The drawing under review shows one solid part. Ordinate dimensions are in mm from its lowest x, y, z. A direction names the side the tool comes from. Coordinates: 2 decimals unless noted, no trailing zeros. Order: outer loops, then holes, each group sorted by start corner. A loop starts at its lowest first (then second) coordinate and runs counter-clockwise, first axis right, second up. Notation, with made-up numbers: (65.5, 40.25) -> (84.5, 40.25) arc R24 ccw to (84.5, 55.25) -> close; hole circle Ø2 at (29.5, 48.5). An arc over 180 degrees is marked (long way). Write item = value, one per line.
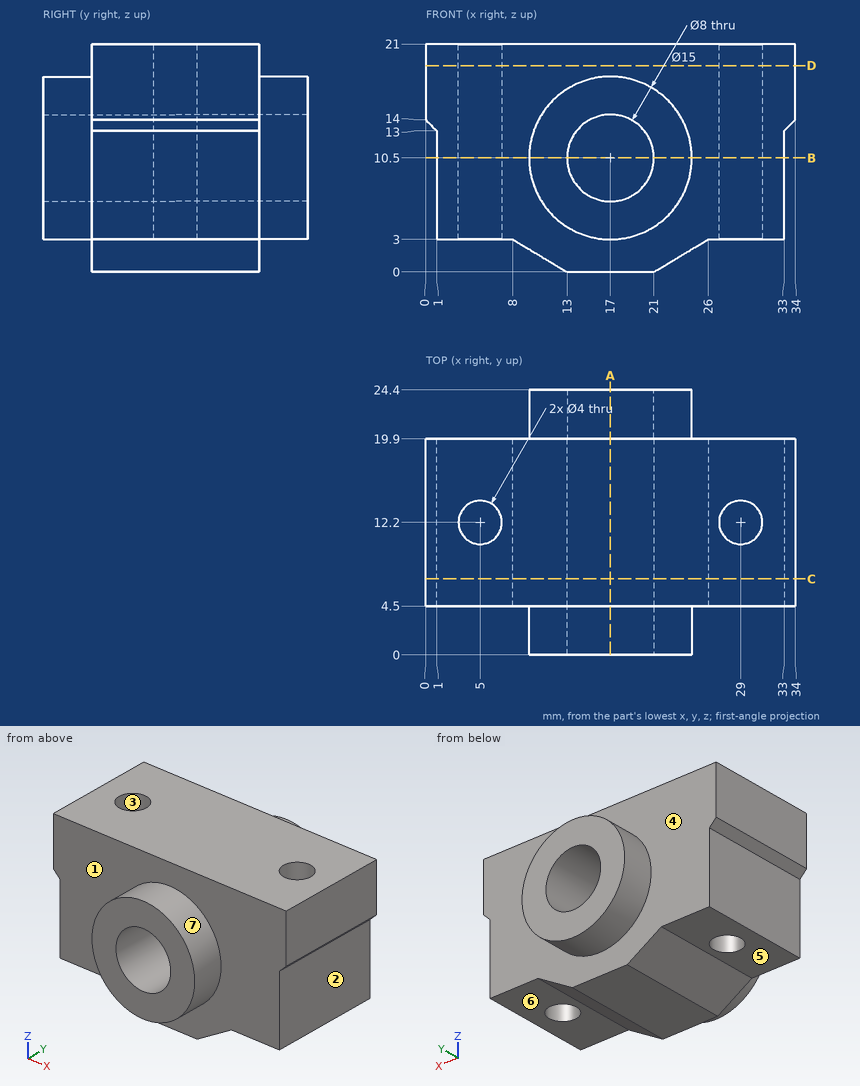
(1) We need section B-B (z = 10.5). Write out the cut boundary in (x, y).
Report:
outline = (1, 4.5) -> (9.5, 4.5) -> (9.5, 0) -> (13, 0) -> (13, 24.4) -> (9.5, 24.4) -> (9.5, 19.9) -> (1, 19.9) -> close; (21, 0) -> (24.5, 0) -> (24.5, 4.5) -> (33, 4.5) -> (33, 19.9) -> (24.5, 19.9) -> (24.5, 24.4) -> (21, 24.4) -> close; hole circle Ø4 at (5, 12.2); hole circle Ø4 at (29, 12.2)
(2) We need section A-A (x = 17). Write out the cut boundary in (y, z), and give its area (3 significant figures).
Report:
outline = (0, 3) -> (4.5, 3) -> (4.5, 0) -> (19.9, 0) -> (19.9, 3) -> (24.4, 3) -> (24.4, 6.5) -> (0, 6.5) -> close; (0, 14.5) -> (24.4, 14.5) -> (24.4, 18) -> (19.9, 18) -> (19.9, 21) -> (4.5, 21) -> (4.5, 18) -> (0, 18) -> close
area = 263 mm²
(3) We need section C-C (y = 7). Write out the cut boundary in (x, z), and give its area (3 significant figures).
Report:
outline = (0, 14) -> (1, 13) -> (1, 3) -> (8, 3) -> (13, 0) -> (21, 0) -> (26, 3) -> (33, 3) -> (33, 13) -> (34, 14) -> (34, 21) -> (0, 21) -> close; hole circle Ø8 at (17, 10.5)
area = 580 mm²
(4) Insertion check: pin 1 (6.5 mm diameter, centred on x = 5, y = 12.2, fed in from -Z); pin 2 (12 mm diameter, centred on x = 3.5, y = 7.5, fed in from -Z); pin 3 (3 mm diameter, centred on y = 11.5, z = 7.5, fed in from +X); pin 4 (3 mm diameter, centred on x = 29, y = 12.2, fed in from -Z). Each pin has a flat end and moves straight along its axis. Give the tip position at first contact, or say it passes through.
Report:
pin_1 = 2.85
pin_2 = 2.1
pin_3 = 33
pin_4 = through
(5) For L1, parallel to X at y = 11.25, z = 19.25; L2, parallel to Y at x = 5, z = 8; L3, parallel to X at y = 6.75, z = 5.25, list the stretches that pass through material, from the lowest coordinate up.
Report:
L1 = 0 to 3.24, 6.76 to 27.24, 30.76 to 34
L2 = 4.5 to 10.2, 14.2 to 19.9
L3 = 1 to 33
(6) For the marked faces 4, 5, 6 and 7, list the 3-axis set-ups (+Z, -Z, +X, -X, +Y, -Y) from which the entire face can be reached by the end or side of a thin tool; tool diameter is ignored.
Report:
face_4 = +Y
face_5 = -Z, -X, +Y, -Y
face_6 = -Z, +X, +Y, -Y
face_7 = -Y
(7) The part is to be moulded in two halves that separate along Y. For the marked faces 1, 2 and 3, say which applies: released by +Y, released by -Y, zero draft, split by the parting line, or undercut.
Report:
face_1 = released by -Y
face_2 = zero draft
face_3 = undercut
(8) We need section D-D (z = 19). Write out the cut boundary in (x, y).
Report:
outline = (0, 4.5) -> (34, 4.5) -> (34, 19.9) -> (0, 19.9) -> close; hole circle Ø4 at (5, 12.2); hole circle Ø4 at (29, 12.2)
